The model under review builds one solid part; all positions refer to its coordinate system, in mm. A direction names the side the tool comes from. Round coordinates to 2 decimals unless told otherwise and drop trailing zeros. Loops run counter-clockwise (first coordinate to the right, second up) from the corner with the lowest first, then second, coordinate; pieces in that order, holes last. Notation, with made-up numbers: (16, -32.5) -> (36, -32.5) arc R17 ccw to (36, -26.5) -> close; hole circle Ø8 at (56, 39). An arc over 180 degrees is marked (long way). Use CSV: the item, a comma, the result in double quotes. Start each with the question number.
```python
from build123d import *

# Parameters (mm, degrees)
F0_W     = 80
F0_H     = 50
F1_DEPTH = 50
F2_W     = 20
F2_H     = 15
F3_DEPTH = 80.001
F4_R     = 18
F5_DEPTH = 15
F7_D     = 8
F8_SIZE  = 10


with BuildPart() as f1:
    # F0 (on Front) → F1 (new body)
    with BuildSketch(Plane.XZ):
        with Locations((0, 25)):
            Rectangle(F0_W, F0_H)
    extrude(amount=F1_DEPTH)

    # F2 (on face) → F3 (cut, through all)
    with BuildSketch(Plane.YZ.offset(40)):
        with Locations((-25, 7.5)):
            Rectangle(F2_W, F2_H)
        Polygon((-5, 50), (-35, 50), (-35, 30), (-15, 30), align=None)
    extrude(amount=-F3_DEPTH, mode=Mode.SUBTRACT)

    # F4 (on face) → F5 (cut, through all)
    with BuildSketch(Plane.XZ.offset(50)):
        with Locations((0, 50)):
            Circle(F4_R)
    extrude(amount=-F5_DEPTH, mode=Mode.SUBTRACT)

    # F7 (through all)
    with Locations(Plane.XZ.offset(50)):
        with Locations((-25, 8), (0, 8), (25, 8)):
            Hole(F7_D / 2)

    # F8
    f8_edges = [f1.edges().sort_by_distance(p)[0] for p in [
        (-40, -42.5, 50),
        (40, -42.5, 50),
    ]]
    chamfer(f8_edges, length=F8_SIZE)


solid = f1.part
```
1. The part is to be moulded in two halves that separate along Z. For faces 5 (the face through (35, -42, 45)), 6 (the face through (1, -35, 2)), 7 (the face through (28.2, -7.4, 5.6)), say which applies: pulls with the +Z half, pulls with the -Z half, needs draft (parallel to the pull), parting line crosses it, or undercut.
2. For faces 1 (the face through (0, -43, 32)), 2 (the face through (1, -25, 15)), 3 (the face through (-35, -42, 45)), 4 (the face through (1, -35, 31)), list the 3-axis set-ups (+Z, -Z, +X, -X, +Y, -Y) from which the entire face can be reached by the end or side of a thin tool; tool diameter is ignored.
3. Take a section at D-D, the plane z = 13.5. Give the boundary of the cut face in (x, y), then the cut area to 3 significant figures.
4. Take a section at A-A, the plane x = -25. Give the boundary of the cut face in (y, z).
5. Take a section at B-B, the plane z = 8. Count the separate pieces of the cut face and the enclosed holes in it, then the cut area to 3 significant figures.
6. For line 1 along Z through (x, y) = (-25, -46); line 2 along Y through (x, z) = (-11, 9); line 3 along X through (y, z) = (-40, 6), list the stretches that pass through material, from the lowest coordinate up. Write a range as from..to.
7. Clearance check with flat-ended pins moving along their axes: P1, Ø8, axis at x = -19.5, y = -29, coming from the -Z side; P2, Ø8, axis at x = 11, z = 43, coming from the -Y side; P3, Ø6.5, axis at x = -25, z = 8, coming from the +Y side; P4, Ø6, axis at x = -16, y = -20.5, coming from the +Z side. State where each tip first meets the part, or that it passes through.
8. Take a section at C-C, the plane y = -44.5. Give the boundary of the cut face in (x, z), then the cut area to 3 significant figures.
Results:
1,face 5,"pulls with the +Z half"
1,face 6,"needs draft"
1,face 7,"undercut"
2,face 1,"+Z, -Y"
2,face 2,"-Z, +X, -X"
2,face 3,"+Z, -X, -Y"
2,face 4,"+Z, +X, -X"
3,outline,"(-40, -50) -> (40, -50) -> (40, -35) -> (-40, -35) -> close; (-40, -15) -> (40, -15) -> (40, 0) -> (-40, 0) -> close"
3,area,"2,400 mm²"
4,outline,"(-50, 0) -> (-35, 0) -> (-35, 4) -> (-50, 4) -> close; (-50, 12) -> (-35, 12) -> (-35, 15) -> (-15, 15) -> (-15, 12) -> (0, 12) -> (0, 50) -> (-5, 50) -> (-15, 30) -> (-35, 30) -> (-35, 50) -> (-50, 50) -> close; (-15, 0) -> (0, 0) -> (0, 4) -> (-15, 4) -> close"
5,separate pieces,"8"
5,enclosed holes,"0"
5,area,"1,680 mm²"
6,line 1,"0..4, 12..50"
6,line 2,"-50..-35, -15..0"
6,line 3,"-40..-28.46, -21.54..-3.46, 3.46..21.54, 28.46..40"
7,P1,"z = 15"
7,P2,"y = -10.5"
7,P3,"through"
7,P4,"z = 30"
8,outline,"(-40, 0) -> (40, 0) -> (40, 40) -> (30, 50) -> (18, 50) arc R18 cw to (-18, 50) -> (-30, 50) -> (-40, 40) -> close; hole circle Ø8 at (-25, 8); hole circle Ø8 at (0, 8); hole circle Ø8 at (25, 8)"
8,area,"3,240 mm²"
